Input: part model. Units: mm. Frame: model coordinates. A direction names the side the tool comes from. Give positions to 0.01 mm unless a question says otherwise; leave off trailing zeros. Order: outer loops, then holes, each group sorted by start corner. A loop starts at its lowest first (then second) coordinate and runs counter-clockwise, first axis right, second up. Notation, with made-up numbers: (77, 10) - (86, 10) arc R25 cw to (86, 33) - close; hole circle Ø4 at (-34.75, 14.25). An arc over 180 degrees is marked (long way). Answer in a Markdown table with one row per item. Add a question column.
1. Section query A-A on x = 0.45. Count the separate pieces of the cut face and the enclosed holes in it, and give its area (3 significant figures).
2. Contact query for flat-ended pins moving along their axis: pin 1 (0.6 mm diameter, centred on x = 0, y = 31, fed in from -Z); pin 2 (1 mm diameter, centred on x = -0.5, y = 2.5, fed in from -Z); pin 3 (0.6 mm diameter, centred on x = 0, z = 8.5, fed in from -Y). Output: stop coordinate, or through.
3. Section query B-B on z = 3. Return loops of the section in (x, y), and give its area (3 significant figures).
4. Section query C-C on y = 23.5. Return loops of the section in (x, z).
5. Access query for faces 1 (the face through (0, -0.9, -14)), 2 (the face through (0.014, 33.249, -19.415)), 3 (the face through (0, 10, -19)). Directions: +Z, -Z, +X, -X, +Y, -Y. A direction counts if a zero-diameter tool reaches every point of the face in a straight line with its end or side. Return the directions, or none.
6. Ray query, line 1 (Z direction, x = -0.3, y = 30); line 2 (Y direction, x = -0.25, z = -10); line 3 (Y direction, x = 0.8, z = -18). Return the intervals inside material, ascending. Write a range as [from, to].
7. Mould query, pull axis Z, two halves, no side actions, for faces 4 (the face through (0, -0.9, -20)), 5 (the face through (-0.014, 3.815, -15.001)), 6 (the face through (0.014, 19.87, 21.384)). Classes: released by +Z, released by -Z, zero draft, split by the parting line, or undercut.
```python
from build123d import *

# Parameters (mm, degrees)
SKETCH1_R           = 1
BASE_SHAPE_DEPTH    = 1
BOTTOM_FILLET_R     = 100
MILLING_FILLETS_R   = 1
MILL_START          = -2
SKETCH17_R          = 0.5
MILL_CUTS_1MM_DEPTH = 2


with BuildPart() as part:
    # Sketch1 → Base shape (new, symmetric)
    with BuildSketch(Plane(origin=(0, 0, 0), x_dir=(0, 0, -1), z_dir=(1, 0, 0))):
        with BuildLine():
            Line((13, 20), (9, 20))
            Line((9, 20), (9, 27.5))
            Line((9, 27.5), (21.5, 27.5))
            Line((21.5, 27.5), (21.5, 30.2))
            Line((21.5, 30.2), (19.7, 30.2))
            Line((19.7, 30.2), (19.7, 28.95))
            Line((19.7, 28.95), (17.5, 28.95))
            Line((17.5, 28.95), (17.5, 33.55))
            Line((17.5, 33.55), (19.7, 33.55))
            Line((19.7, 33.55), (19.7, 32.3))
            Line((19.7, 32.3), (21.5, 32.3))
            Line((21.5, 32.3), (21.5, 35))
            Line((21.5, 35), (-8.44638615, 35))
            ThreePointArc((-8.44638615, 35), (-9.003752396, 34.937076705), (-9.533061586, 34.751474294))
            ThreePointArc((-9.533061586, 34.751474294), (-21.444501682, 19.597102087), (-16.791629001, 0.891803961))
            ThreePointArc((-16.791629001, 0.891803961), (-15.933367715, 0.233892092), (-14.877548152, 0))
            Line((-14.877548152, 0), (-14.996910346, 0))
            Line((-14.996910346, 0), (5.9, -2))
            Line((5.9, -2), (10.9, -2))
            Line((10.9, -2), (10.9, 0))
            Line((10.9, 0), (13, 0))
            Line((13, 0), (13, -0.9))
            Line((13, -0.9), (15.95, -0.9))
            Line((15.95, -0.9), (15.95, 1.9))
            Line((15.95, 1.9), (14.7, 1.9))
            Line((14.7, 1.9), (14.7, 4.1))
            Line((14.7, 4.1), (19.3, 4.1))
            Line((19.3, 4.1), (19.3, 1.9))
            Line((19.3, 1.9), (18.05, 1.9))
            Line((18.05, 1.9), (18.05, -0.9))
            Line((18.05, -0.9), (21, -0.9))
            Line((21, -0.9), (21, 5))
            Line((21, 5), (19, 5))
            Line((19, 5), (19, 15))
            Line((19, 15), (21, 15))
            Line((21, 15), (21, 20.9))
            Line((21, 20.9), (18.05, 20.9))
            Line((18.05, 20.9), (18.05, 19.1))
            Line((18.05, 19.1), (19.3, 19.1))
            Line((19.3, 19.1), (19.3, 16.9))
            Line((19.3, 16.9), (14.7, 16.9))
            Line((14.7, 16.9), (14.7, 19.1))
            Line((14.7, 19.1), (15.95, 19.1))
            Line((15.95, 19.1), (15.95, 20.9))
            Line((15.95, 20.9), (13, 20.9))
            Line((13, 20.9), (13, 20))
        make_face()
        with BuildLine():
            ThreePointArc((-0.868240859, 10.07596123), (-0.05708131, 8.91750532), (-1.215537181, 8.106345718))
            ThreePointArc((-1.215537181, 8.106345718), (-3.232240261, 8.790924151), (-4.949747462, 10.050252526))
            ThreePointArc((-4.949747462, 10.050252526), (-4.949747471, 11.464466091), (-3.535533905, 11.464466093))
            ThreePointArc((-3.535533905, 11.464466093), (-2.308743052, 10.564945827), (-0.868240859, 10.07596123))
        make_face(mode=Mode.SUBTRACT)
        with Locations((-4.5, 15)):
            Circle(SKETCH1_R, mode=Mode.SUBTRACT)
        with Locations((-9, 15)):
            Circle(SKETCH1_R, mode=Mode.SUBTRACT)
        with Locations((-3, 32.5)):
            Circle(SKETCH1_R, mode=Mode.SUBTRACT)
        with Locations((0, 15)):
            Circle(SKETCH1_R, mode=Mode.SUBTRACT)
        with Locations((-14.877548152, 2.5)):
            Circle(SKETCH1_R, mode=Mode.SUBTRACT)
        with BuildLine():
            Line((-9, 33.5), (-7, 33.5))
            ThreePointArc((-7, 33.5), (-6, 32.5), (-7, 31.5))
            Line((-7, 31.5), (-9, 31.5))
            ThreePointArc((-9, 31.5), (-10, 32.5), (-9, 33.5))
        make_face(mode=Mode.SUBTRACT)
    extrude(amount=BASE_SHAPE_DEPTH, both=True)

    # Bottom fillet
    # the kernel refuses this fillet: 100 mm, written as the material it takes off along each edge
    with BuildSketch(Plane(origin=(-12.9362194, -2, -5.9), x_dir=(0, 0, -1), z_dir=(1, 0, 0))) as bottom_fillet_piece_1:
        with BuildLine():
            CenterArc((BOTTOM_FILLET_R * 0.0477448775998, BOTTOM_FILLET_R), BOTTOM_FILLET_R, 264.532991667, 5.467008333)
            Line((-BOTTOM_FILLET_R * 0.0475276967795, BOTTOM_FILLET_R * 0.00454877740235), (0, 0))
            Line((0, 0), (BOTTOM_FILLET_R * 0.0477448775998, 0))
        make_face()
    extrude(amount=25.8724388, mode=Mode.SUBTRACT)

    # Milling fillets
    milling_fillets_edges = [part.edges().sort_by_distance(p)[0] for p in [
        (0, 33.55, -19.7),
        (0, 33.55, -17.5),
        (0, 28.95, -17.5),
        (0, 28.95, -19.7),
        (0, 27.5, -9),
        (0, 19.1, -14.7),
        (0, 16.9, -14.7),
        (0, 16.9, -19.3),
        (0, 19.1, -19.3),
        (0, 15, -19),
        (0, 5, -19),
        (0, 1.9, -19.3),
        (0, 4.1, -19.3),
        (0, 4.1, -14.7),
        (0, 1.9, -14.7),
    ]]
    fillet(milling_fillets_edges, radius=MILLING_FILLETS_R)

    # Sketch17 → Mill cuts 1mm (cut)
    with BuildSketch(Plane(origin=(1, 0, 0), x_dir=(0, 0, -1), z_dir=(1, 0, 0)).offset(MILL_START)):
        with Locations((9.353553391, 20.353553391)):
            Circle(SKETCH17_R)
        with Locations((12.646446609, 20.353553391)):
            Circle(SKETCH17_R)
        with Locations((12.646446609, -0.353553391)):
            Circle(SKETCH17_R)
        with Locations((11.253553391, -0.353553391)):
            Circle(SKETCH17_R)
    extrude(amount=MILL_CUTS_1MM_DEPTH, mode=Mode.SUBTRACT)


solid = part.part
```
Answer:
| question | item | result |
|---|---|---|
| 1 | separate pieces | 1 |
| 1 | enclosed holes | 7 |
| 1 | area | 1,270 mm² |
| 2 | pin 1 | stops at z = -17.5 |
| 2 | pin 2 | stops at z = -21 |
| 2 | pin 3 | stops at y = -0.65 |
| 3 | outline | (-1, -1.15) - (1, -1.15) - (1, 8.68) - (-1, 8.68) - close; (-1, 11) - (1, 11) - (1, 31.5) - (-1, 31.5) - close; (-1, 33.5) - (1, 33.5) - (1, 35) - (-1, 35) - close |
| 3 | area | 63.6 mm² |
| 4 | outline | (-1, -9) - (1, -9) - (1, 20.22) - (-1, 20.22) - close |
| 5 | face 1 | -Z, +X, -X, -Y |
| 5 | face 2 | +X, -X |
| 5 | face 3 | -Z, +X, -X |
| 6 | line 1 | z = [-21.5, -19.7], [-17.5, 16] |
| 6 | line 2 | y = [-2, 20], [27.5, 35] |
| 6 | line 3 | y = [4.1, 16.9], [27.5, 29.08], [33.42, 35] |
| 7 | face 4 | zero draft |
| 7 | face 5 | undercut |
| 7 | face 6 | released by +Z |
